```python
from build123d import *

# Parameters (mm, degrees)
F1_DEPTH = 6.42
F2_R     = 4.76
F3_DEPTH = 34
F4_R     = 4.76
F5_DEPTH = 18.2
F7_DEPTH = 18.2


with BuildPart() as f1:
    # F0 (on Top) → F1 (new body)
    with BuildSketch(Plane.XY):
        with BuildLine():
            Line((16.5, 7.4), (-16.5, 7.4))
            ThreePointArc((-16.5, 7.4), (-23.9, 0), (-16.5, -7.4))
            Line((-16.5, -7.4), (16.5, -7.4))
            ThreePointArc((16.5, -7.4), (23.9, 0), (16.5, 7.4))
        make_face()
    extrude(amount=F1_DEPTH)

    # F2 (on face) → F3 (join)
    with BuildSketch(Plane(origin=(0, 0, 0), x_dir=(1, 0, 0), z_dir=(0, 0, -1))):
        Circle(F2_R)
    extrude(amount=F3_DEPTH)

    # F4 (on face) → F5 (join)
    with BuildSketch(Plane.XY.offset(6.42)):
        Circle(F4_R)
    extrude(amount=F5_DEPTH)

    # F6 (on face) → F7 (join)
    with BuildSketch(Plane.XY.offset(24.62)):
        with BuildLine():
            ThreePointArc((-3.247645, -3.48), (-1.745394, -4.428453), (0, -4.76))
            Line((0, -4.76), (0, -3.48))
            Line((0, -3.48), (-3.247645, -3.48))
        make_face()
        with BuildLine():
            Line((0, -3.48), (0, -4.76))
            ThreePointArc((0, -4.76), (1.745394, -4.428453), (3.247645, -3.48))
            Line((3.247645, -3.48), (0, -3.48))
        make_face()
    extrude(amount=-F7_DEPTH)


solid = f1.part
```
For this review, take the finished solid that the model builds, in its own axes (mm). A direction names the side the tool comes from. Give positions to 0.01 mm unless a question says otherwise; leave off trailing zeros. Write each loop counter-clockwise with the first axis right and the second up, starting at its lowest first coordinate (ties: lowest second). Pieces come first, ordered by that corner, then holes.
Item 1: Take a section at A-A (y = 0). Give the boundary of the cut face in (x, z), and give its area (3 significant figures).
Item 2: Take a section at B-B (x = 11). Give the boundary of the cut face in (y, z), and give its area (3 significant figures).
Item 3: Insertion check: P1, Ø8, axis at y = 5.5, z = -19, coming from the +X side; P2, Ø5, axis at y = 5.5, z = -23, coming from the +X side; P3, Ø5, axis at y = -3.5, z = -9.5, coming from the +X side. Each pin has a flat end and moves straight along its axis. Give the tip position at first contact, or say it passes through.
Item 4: Wall thickness on probe 1 along Z at (x, y) = (-13, 4.5); probe 2 along X at (y, z) = (0, 10); probe 3 along X at (y, z) = (2.25, -9.5): over which ranges is each line inside the solid? List them lowest first.
Item 5: Take a section at C-C (z = -1.5). Give the boundary of the cut face in (x, y), and give its area (3 significant figures).
Item 6: Machinability: for faces 1 (the face through (0, -7.4, 3)), 2 (the face through (-1.032, 4.647, -16.762)), which of the approach directions +Z, -Z, +X, -X, +Y, -Y give a long, thin tool a straight path to every point of the face, cutting with its end or side? Answer none if there is none.
Item 7: Take a section at D-D (x = 19). Give the boundary of the cut face in (y, z).
Established:
1. outline: (-23.9, 0) - (-4.76, 0) - (-4.76, -34) - (4.76, -34) - (4.76, 0) - (23.9, 0) - (23.9, 6.42) - (4.76, 6.42) - (4.76, 24.62) - (-4.76, 24.62) - (-4.76, 6.42) - (-23.9, 6.42) - close
1. area: 804 mm2
2. outline: (-7.4, 0) - (7.4, 0) - (7.4, 6.42) - (-7.4, 6.42) - close
2. area: 95.0 mm2
3. P1: stops at x = 4.52
3. P2: stops at x = 3.7
3. P3: stops at x = 4.65
4. probe 1: z = 0 to 6.42
4. probe 2: x = -4.76 to 4.76
4. probe 3: x = -4.19 to 4.19
5. outline: circle Ø9.52 at (0, 0)
5. area: 71.2 mm2
6. face 1: +Z, -Z, +X, -X, -Y
6. face 2: -Z
7. outline: (-6.96, 0) - (6.96, 0) - (6.96, 6.42) - (-6.96, 6.42) - close
